Geometry: see drawing. Coordinates: mm, zero at the bounding-box minimum. A direction names the side the tool comes from. Coordinates: 2 decimals unless noted, no trailing zeros. Write each loop counter-clockwise with the first axis right and the second up, starting at its lowest first coordinate (ties: lowest second). Pieces come first, ordered by that corner, then holes.
1) Set-up query: the marked faces 1 and 2. Return all of +Z, -Z, +X, -X, +Y, -Y with unobstructed straight access to the full face (end or side cutting, diameter ignored); none if empty.
2) Line query: L1, parallel to Z at x = 2.65, y = 1.4; L2, parallel to Z at x = 1.5, y = 4.25; L3, parallel to X at y = 1.9, z = 1. Output: solid intervals per line, ascending.
3) Section query B-B (z = 4). Output: boundary loops of the cut face in (x, y).
4) Draft query along X for the marked faces 3, 4 and 5. Return one class per face: pulls with the +X half, pulls with the -X half, needs draft (parallel to the pull), parting line crosses it, or undercut.
5) Section query C-C (x = 3). Output: boundary loops of the cut face in (y, z).
6) Section query D-D (z = 2). Output: boundary loops of the cut face in (x, y).
7) Pin query (flat end, axial travel): pin 1 Ø1 at (x, z) = (3, 8.5) entering from -Y; pin 2 Ø1.5 at (y, z) = (1, 2) entering from +X. Return the tip coordinate at first contact, or that it passes through.
8) Section query A-A (y = 2.25). Output: boundary loops of the cut face in (x, z), then the cut area to 3 significant figures.
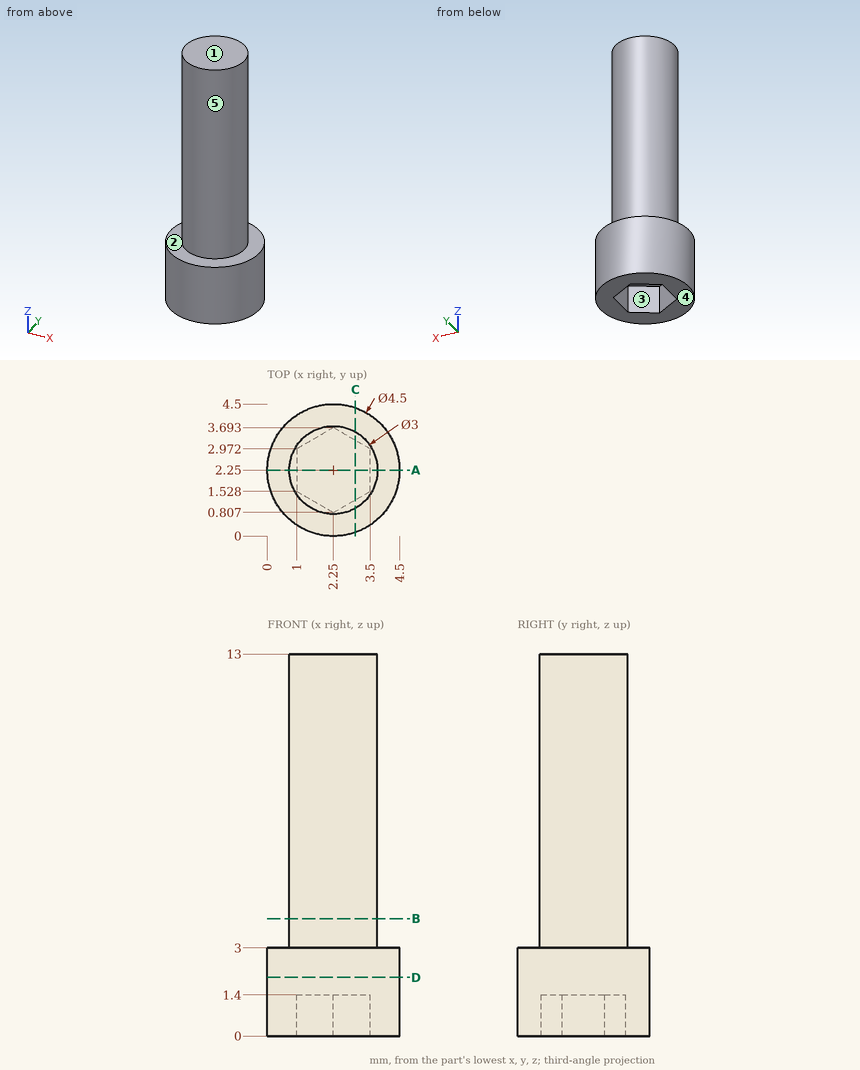
Answer:
1. face 1: +Z, +X, -X, +Y, -Y
1. face 2: +Z
2. L1: z = 1.4 to 13
2. L2: z = 0 to 3
2. L3: x = 0.03 to 1, 3.5 to 4.47
3. outline: circle Ø3 at (2.25, 2.25)
4. face 3: undercut
4. face 4: needs draft
4. face 5: parting line crosses it
5. outline: (0.13, 0) - (1.24, 0) - (1.24, 1.4) - (3.26, 1.4) - (3.26, 0) - (4.37, 0) - (4.37, 3) - (3.55, 3) - (3.55, 13) - (0.95, 13) - (0.95, 3) - (0.13, 3) - close
6. outline: circle Ø4.5 at (2.25, 2.25)
7. pin 1: stops at y = 0.77
7. pin 2: stops at x = 4.44
8. outline: (0, 0) - (1, 0) - (1, 1.4) - (3.5, 1.4) - (3.5, 0) - (4.5, 0) - (4.5, 3) - (3.75, 3) - (3.75, 13) - (0.75, 13) - (0.75, 3) - (0, 3) - close
8. area: 40.0 mm2
